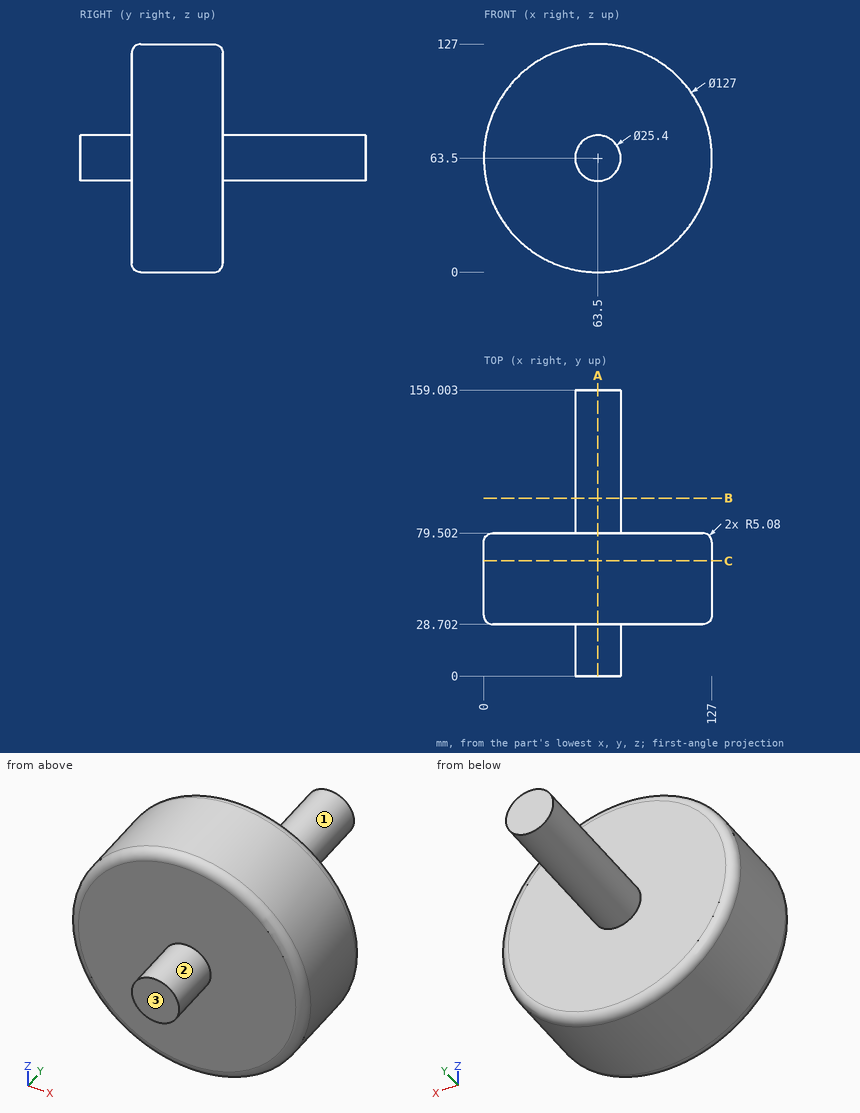
For this review, use the dimensioned drawing (mm, ordinates from the lowest corner) and the shaded views. A direction names the side the tool comes from. Coordinates: 2 decimals unless noted, no trailing zeros. Write each loop counter-clockwise with the first axis right and the second up, starting at its lowest first coordinate (ties: lowest second). Pieces come first, ordered by that corner, then holes. Notation, with made-up numbers: (10.5, 23.5) -> (47.5, 23.5) arc R11 ccw to (47.5, 42.5) -> close; hole circle Ø11 at (14.25, -5). An arc over 180 degrees is marked (long way). Put each result on its own line as item: value.
Q1. Take a section at A-A, the plane x = 63.5. State the section outline as (y, z) points.
From the geometry:
outline: (0, 50.8) -> (28.7, 50.8) -> (28.7, 5.08) arc R5.08 ccw to (33.78, 0) -> (74.42, 0) arc R5.08 ccw to (79.5, 5.08) -> (79.5, 50.8) -> (159, 50.8) -> (159, 76.2) -> (79.5, 76.2) -> (79.5, 121.92) arc R5.08 ccw to (74.42, 127) -> (33.78, 127) arc R5.08 ccw to (28.7, 121.92) -> (28.7, 76.2) -> (0, 76.2) -> close
Q2. Clearance check with flat-ended pins moving along their axes: pin 1 Ø6 at (y, z) = (119.5, 49) entering from +X; pin 2 Ø5 at (x, y) = (27, 71.5) entering from +Z; pin 3 Ø5 at (x, y) = (74, 37.5) entering from -Z. State where each tip first meets the part, or that it passes through.
From the geometry:
pin 1: stops at x = 68.89
pin 2: stops at z = 117.13
pin 3: stops at z = 0.51
Q3. Tool access review of the marked faces 1, 2 and 3: name each direction out of +Z, -Z, +X, -X, +Y, -Y from which nothing blocks a thin tool from reaching the whole face with its end or side.
From the geometry:
face 1: +Y
face 2: -Y
face 3: +Z, -Z, +X, -X, -Y
Q4. Wall thickness on L1, parallel to Y at x = 54, z = 12.5; L2, parallel to Z at x = 70, y = 113.5; L3, parallel to Z at x = 79, y = 30 (1 decimal): over which ranges is each line inside the solid? List them lowest first.
From the geometry:
L1: y = 28.7 to 79.5
L2: z = 52.59 to 74.41
L3: z = 3.7 to 123.3
Q5. Take a section at B-B, the plane y = 99. State the section outline as (x, z) points.
From the geometry:
outline: circle Ø25.4 at (63.5, 63.5)
Q6. Take a section at C-C, the plane y = 64. State the section outline as (x, z) points.
From the geometry:
outline: circle Ø127 at (63.5, 63.5)
